from build123d import *

# Parameters (mm, degrees)
F1_DEPTH  = 50.8
F2_R      = 14.9225
F3_DEPTH  = 15.9385
F4_R      = 2.54
F5_DEPTH  = 25.401
F6_R      = 1.190625
F7_DEPTH  = 25.401
F8_R      = 1.190625
F9_DEPTH  = 25.401
F10_R     = 2.0193
F11_DEPTH = 6.35
F13_DEPTH = 4.1275
F14_R     = 1.5875
F15_DEPTH = 50.801


with BuildPart() as f1:
    # F0 (on Front) → F1 (new body)
    with BuildSketch(Plane.XZ):
        with BuildLine():
            Line((-29.972, 0), (-44.45, 0))
            Line((-44.45, 0), (-44.45, -25.4))
            Line((-44.45, -25.4), (44.45, -25.4))
            Line((44.45, -25.4), (44.45, 0))
            Line((44.45, 0), (29.972, 0))
            ThreePointArc((29.972, 0), (19.05, -10.922), (8.128, 0))
            Line((8.128, 0), (-8.128, 0))
            ThreePointArc((-8.128, 0), (-19.05, -10.922), (-29.972, 0))
        make_face()
    extrude(amount=F1_DEPTH)

    # F2 (on face) → F3 (cut)
    with BuildSketch(Plane.XZ.offset(50.8)):
        with Locations((-19.05, 0)):
            Circle(F2_R)
        with Locations((19.05, 0)):
            Circle(F2_R)
    extrude(amount=-F3_DEPTH, mode=Mode.SUBTRACT)

    # F4 (on face) → F5 (cut, through all)
    with BuildSketch(Plane(origin=(0, 0, -25.4), x_dir=(1, 0, 0), z_dir=(0, 0, -1))):
        with Locations((-38.1, 44.45)):
            Circle(F4_R)
        with Locations((0, 44.45)):
            Circle(F4_R)
        with Locations((38.1, 44.45)):
            Circle(F4_R)
        with Locations((38.1, 6.35)):
            Circle(F4_R)
        with Locations((0, 6.35)):
            Circle(F4_R)
        with Locations((-38.1, 6.35)):
            Circle(F4_R)
    extrude(amount=-F5_DEPTH, mode=Mode.SUBTRACT)

    # F6 (on face) → F7 (cut, through all)
    with BuildSketch(Plane.XY):
        with Locations((37.211, -25.4)):
            Circle(F6_R)
    extrude(amount=-F7_DEPTH, mode=Mode.SUBTRACT)

    # F8 (on face) → F9 (cut, through all)
    with BuildSketch(Plane.XY):
        with Locations((-37.211, -25.4)):
            Circle(F8_R)
    extrude(amount=-F9_DEPTH, mode=Mode.SUBTRACT)

    # F10 (on face) + F8 (on face) → F11 (cut)
    with BuildSketch(Plane(origin=(0, 0, -25.4), x_dir=(1, 0, 0), z_dir=(0, 0, -1))):
        with Locations((-19.05, 6.35)):
            Circle(F10_R)
        with Locations((-19.05, 44.45)):
            Circle(F10_R)
        with Locations((19.05, 44.45)):
            Circle(F10_R)
        with Locations((19.05, 6.35)):
            Circle(F10_R)
    with BuildSketch(Plane.XY):
        with Locations((-37.211, -25.4)):
            Circle(F8_R)
    extrude(amount=-F11_DEPTH, mode=Mode.SUBTRACT)

    # F12 (on face) → F13 (cut)
    with BuildSketch(Plane(origin=(0, 0, -25.4), x_dir=(1, 0, 0), z_dir=(0, 0, -1))):
        with BuildLine():
            Line((-35.808641, 49.2125), (-40.391359, 49.2125))
            ThreePointArc((-40.391359, 49.2125), (-40.788234, 49.106158), (-41.078767, 48.815625))
            Line((-41.078767, 48.815625), (-43.370125, 44.846875))
            ThreePointArc((-43.370125, 44.846875), (-43.476468, 44.45), (-43.370125, 44.053125))
            Line((-43.370125, 44.053125), (-41.078767, 40.084375))
            ThreePointArc((-41.078767, 40.084375), (-40.788234, 39.793842), (-40.391359, 39.6875))
            Line((-40.391359, 39.6875), (-35.808641, 39.6875))
            ThreePointArc((-35.808641, 39.6875), (-35.411766, 39.793842), (-35.121233, 40.084375))
            Line((-35.121233, 40.084375), (-32.829875, 44.053125))
            ThreePointArc((-32.829875, 44.053125), (-32.723532, 44.45), (-32.829875, 44.846875))
            Line((-32.829875, 44.846875), (-35.121233, 48.815625))
            ThreePointArc((-35.121233, 48.815625), (-35.411766, 49.106158), (-35.808641, 49.2125))
        make_face()
        Polygon((2.749631, 49.2125), (-2.749631, 49.2125), (-5.499261, 44.45), (-2.749631, 39.6875), (2.749631, 39.6875), (5.499261, 44.45), align=None)
        Polygon((40.849631, 49.2125), (35.350369, 49.2125), (32.600739, 44.45), (35.350369, 39.6875), (40.849631, 39.6875), (43.599261, 44.45), align=None)
        Polygon((40.849631, 11.1125), (35.350369, 11.1125), (32.600739, 6.35), (35.350369, 1.5875), (40.849631, 1.5875), (43.599261, 6.35), align=None)
        Polygon((2.749631, 11.1125), (-2.749631, 11.1125), (-5.499261, 6.35), (-2.749631, 1.5875), (2.749631, 1.5875), (5.499261, 6.35), align=None)
        Polygon((-35.350369, 11.1125), (-40.849631, 11.1125), (-43.599261, 6.35), (-40.849631, 1.5875), (-35.350369, 1.5875), (-32.600739, 6.35), align=None)
    extrude(amount=-F13_DEPTH, mode=Mode.SUBTRACT)

    # F14 (on face) → F15 (cut, through all)
    with BuildSketch(Plane.XZ.offset(50.8)):
        with Locations((29.976631, -15.604846)):
            Circle(F14_R)
        with Locations((8.123369, -15.604846)):
            Circle(F14_R)
        with Locations((-8.123369, -15.604846)):
            Circle(F14_R)
        with Locations((-29.976631, -15.604846)):
            Circle(F14_R)
    extrude(amount=-F15_DEPTH, mode=Mode.SUBTRACT)


solid = f1.part
Check sheet for the modelled part. Datum: model origin and axes. Units: mm. A direction names the side the tool comes from. Give positions to 0.01 mm unless a question says otherwise; leave off trailing zeros. Order: outer loops, then holes, each group sorted by start corner. A loop starts at its lowest first (then second) coordinate and runs counter-clockwise, first axis right, second up. Notation, with made-up numbers: (86, 78) - (104, 78) arc R33 ccw to (104, 106) - close; hole circle Ø11 at (27, 61.25). An arc over 180 degrees is marked (long way). Answer as CSV lines item,"result".
1. Section check B-B (y = -29). State how many separate pieces and enclosed holes the cut face has, then the cut area to 3 significant figures.
Result sheet:
separate pieces,"1"
enclosed holes,"4"
area,"1,850 mm²"
2. Mould release check, pull along Z, two halves, no side actions. Record for faces 3 (the face through (31.49, -25.76, -15.13)), 4 (the face through (42.21, -42.04, -23.37)), 5 (the face through (-41, -43, -21.272)), 6 (the face through (-9.71, -25.76, -15.54)): released by +Z, released by -Z, zero draft, split by the parting line, or undercut.
Result sheet:
face 3,"undercut"
face 4,"zero draft"
face 5,"released by -Z"
face 6,"undercut"
3. Tool access check on faces 1 (the face through (-1, -9, -21.272)), 2 (the face through (36.23, -46.17, -10.79)). Record the directions out of +Z, -Z, +X, -X, +Y, -Y that give a thin tool (end or side, any length) a straight path to the whole face; none if there is none.
Result sheet:
face 1,"-Z"
face 2,"+Z, -Z"
4. Go/stop test with flat-tipped pins: P1, Ø2.5, axis at x = 29.98, z = -15.6, coming from the +Y side; P2, Ø10, axis at x = -18, y = -5.5, coming from the +Z side; P3, Ø5, axis at x = -39.5, y = -42.5, coming from the -Z side; P4, Ø6, axis at x = -20.5, z = -10, coming from the -Y side. Record where each tip stops, or that it passes through.
Result sheet:
P1,"through"
P2,"z = -9.09"
P3,"z = -21.27"
P4,"y = -34.86"
5. Section check C-C (x = 19.05). Record the boundary of the cut face in (y, z).
Result sheet:
outline,"(-50.8, -25.4) - (-46.47, -25.4) - (-46.47, -19.05) - (-42.43, -19.05) - (-42.43, -25.4) - (-8.37, -25.4) - (-8.37, -19.05) - (-4.33, -19.05) - (-4.33, -25.4) - (0, -25.4) - (0, -10.92) - (-34.86, -10.92) - (-34.86, -14.92) - (-50.8, -14.92) - close"
6. Scan lines: probe 1 along Y at (x, z) = (0, -5.5); probe 2 along X at (y, z) = (-44.5, -21.5); probe 3 along X at (y, z) = (-17, -8). Record each from-to range of solid material in increasing order. Write a range as from..to.
Result sheet:
probe 1,"-50.8..-46.99, -41.91..-8.89, -3.81..0"
probe 2,"-44.45..-43.47, -32.73..-21.07, -17.03..-5.47, 5.47..17.03, 21.07..32.63, 43.57..44.45"
probe 3,"-44.45..-26.49, -11.61..11.61, 26.49..44.45"
7. Section check A-A (x = 0). Record the boundary of the cut face in (y, z), then the cut area to 3 significant figures.
Result sheet:
outline,"(-50.8, -25.4) - (-49.21, -25.4) - (-49.21, -21.27) - (-46.99, -21.27) - (-46.99, 0) - (-50.8, 0) - close; (-41.91, -21.27) - (-39.69, -21.27) - (-39.69, -25.4) - (-11.11, -25.4) - (-11.11, -21.27) - (-8.89, -21.27) - (-8.89, 0) - (-41.91, 0) - close; (-3.81, -21.27) - (-1.59, -21.27) - (-1.59, -25.4) - (0, -25.4) - (0, 0) - (-3.81, 0) - close"
area,"996 mm²"
